from build123d import *

# Parameters (mm, degrees)
SKETCH1_W           = 152.4
SKETCH1_H           = 254
BOSS_EXTRUDE1_DEPTH = 6.35
CUT_EXTRUDE2_REACH  = 150.242
SKETCH3_R           = 2.5
CUT_EXTRUDE3_REACH  = 150.242
SKETCH4_R           = 2.75


with BuildPart() as part:
    # Sketch1 → Boss-Extrude1 (new body)
    with BuildSketch(Plane.XY):
        Rectangle(SKETCH1_W, SKETCH1_H)
    extrude(amount=BOSS_EXTRUDE1_DEPTH)

    # Sketch3 → Cut-Extrude2 (cut, up to next)
    with BuildSketch(Plane(origin=(0, 0, 0), x_dir=(-1, 0, 0), z_dir=(0, 0, -1)), mode=Mode.PRIVATE) as cut_extrude2_sk1:
        with Locations((63.7, -20.45)):
            Circle(SKETCH3_R)
    cut_extrude2_tool1 = extrude(cut_extrude2_sk1.sketch, amount=-CUT_EXTRUDE2_REACH, mode=Mode.PRIVATE) & part.part
    # Sketch3 → Cut-Extrude2 (cut, up to next)
    with BuildSketch(Plane(origin=(0, 0, 0), x_dir=(-1, 0, 0), z_dir=(0, 0, -1)), mode=Mode.PRIVATE) as cut_extrude2_sk2:
        with Locations((38.7, -20.45)):
            Circle(SKETCH3_R)
    cut_extrude2_tool2 = extrude(cut_extrude2_sk2.sketch, amount=-CUT_EXTRUDE2_REACH, mode=Mode.PRIVATE) & part.part
    # Sketch3 → Cut-Extrude2 (cut, up to next)
    with BuildSketch(Plane(origin=(0, 0, 0), x_dir=(-1, 0, 0), z_dir=(0, 0, -1)), mode=Mode.PRIVATE) as cut_extrude2_sk3:
        with Locations((38.7, -45.45)):
            Circle(SKETCH3_R)
    cut_extrude2_tool3 = extrude(cut_extrude2_sk3.sketch, amount=-CUT_EXTRUDE2_REACH, mode=Mode.PRIVATE) & part.part
    # Sketch3 → Cut-Extrude2 (cut, up to next)
    with BuildSketch(Plane(origin=(0, 0, 0), x_dir=(-1, 0, 0), z_dir=(0, 0, -1)), mode=Mode.PRIVATE) as cut_extrude2_sk4:
        with Locations((63.7, -45.45)):
            Circle(SKETCH3_R)
    cut_extrude2_tool4 = extrude(cut_extrude2_sk4.sketch, amount=-CUT_EXTRUDE2_REACH, mode=Mode.PRIVATE) & part.part
    # Sketch3 → Cut-Extrude2 (cut, up to next)
    with BuildSketch(Plane(origin=(0, 0, 0), x_dir=(-1, 0, 0), z_dir=(0, 0, -1)), mode=Mode.PRIVATE) as cut_extrude2_sk5:
        with Locations((63.7, -70.45)):
            Circle(SKETCH3_R)
    cut_extrude2_tool5 = extrude(cut_extrude2_sk5.sketch, amount=-CUT_EXTRUDE2_REACH, mode=Mode.PRIVATE) & part.part
    # Sketch3 → Cut-Extrude2 (cut, up to next)
    with BuildSketch(Plane(origin=(0, 0, 0), x_dir=(-1, 0, 0), z_dir=(0, 0, -1)), mode=Mode.PRIVATE) as cut_extrude2_sk6:
        with Locations((38.7, -70.45)):
            Circle(SKETCH3_R)
    cut_extrude2_tool6 = extrude(cut_extrude2_sk6.sketch, amount=-CUT_EXTRUDE2_REACH, mode=Mode.PRIVATE) & part.part
    # Sketch3 → Cut-Extrude2 (cut, up to next)
    with BuildSketch(Plane(origin=(0, 0, 0), x_dir=(-1, 0, 0), z_dir=(0, 0, -1)), mode=Mode.PRIVATE) as cut_extrude2_sk7:
        with Locations((38.7, -95.45)):
            Circle(SKETCH3_R)
    cut_extrude2_tool7 = extrude(cut_extrude2_sk7.sketch, amount=-CUT_EXTRUDE2_REACH, mode=Mode.PRIVATE) & part.part
    # Sketch3 → Cut-Extrude2 (cut, up to next)
    with BuildSketch(Plane(origin=(0, 0, 0), x_dir=(-1, 0, 0), z_dir=(0, 0, -1)), mode=Mode.PRIVATE) as cut_extrude2_sk8:
        with Locations((63.7, -95.45)):
            Circle(SKETCH3_R)
    cut_extrude2_tool8 = extrude(cut_extrude2_sk8.sketch, amount=-CUT_EXTRUDE2_REACH, mode=Mode.PRIVATE) & part.part
    # Sketch3 → Cut-Extrude2 (cut, up to next)
    with BuildSketch(Plane(origin=(0, 0, 0), x_dir=(-1, 0, 0), z_dir=(0, 0, -1)), mode=Mode.PRIVATE) as cut_extrude2_sk9:
        with Locations((-11.738, -61.16)):
            Circle(SKETCH3_R)
    cut_extrude2_tool9 = extrude(cut_extrude2_sk9.sketch, amount=-CUT_EXTRUDE2_REACH, mode=Mode.PRIVATE) & part.part
    # Sketch3 → Cut-Extrude2 (cut, up to next)
    with BuildSketch(Plane(origin=(0, 0, 0), x_dir=(-1, 0, 0), z_dir=(0, 0, -1)), mode=Mode.PRIVATE) as cut_extrude2_sk10:
        with Locations((-11.738, -36.16)):
            Circle(SKETCH3_R)
    cut_extrude2_tool10 = extrude(cut_extrude2_sk10.sketch, amount=-CUT_EXTRUDE2_REACH, mode=Mode.PRIVATE) & part.part
    # Sketch3 → Cut-Extrude2 (cut, up to next)
    with BuildSketch(Plane(origin=(0, 0, 0), x_dir=(-1, 0, 0), z_dir=(0, 0, -1)), mode=Mode.PRIVATE) as cut_extrude2_sk11:
        with Locations((-36.738, -61.16)):
            Circle(SKETCH3_R)
    cut_extrude2_tool11 = extrude(cut_extrude2_sk11.sketch, amount=-CUT_EXTRUDE2_REACH, mode=Mode.PRIVATE) & part.part
    # Sketch3 → Cut-Extrude2 (cut, up to next)
    with BuildSketch(Plane(origin=(0, 0, 0), x_dir=(-1, 0, 0), z_dir=(0, 0, -1)), mode=Mode.PRIVATE) as cut_extrude2_sk12:
        with Locations((-36.738, -36.16)):
            Circle(SKETCH3_R)
    cut_extrude2_tool12 = extrude(cut_extrude2_sk12.sketch, amount=-CUT_EXTRUDE2_REACH, mode=Mode.PRIVATE) & part.part
    # Sketch3 → Cut-Extrude2 (cut, up to next)
    with BuildSketch(Plane(origin=(0, 0, 0), x_dir=(-1, 0, 0), z_dir=(0, 0, -1)), mode=Mode.PRIVATE) as cut_extrude2_sk13:
        with Locations((-11.738, -11.16)):
            Circle(SKETCH3_R)
    cut_extrude2_tool13 = extrude(cut_extrude2_sk13.sketch, amount=-CUT_EXTRUDE2_REACH, mode=Mode.PRIVATE) & part.part
    # Sketch3 → Cut-Extrude2 (cut, up to next)
    with BuildSketch(Plane(origin=(0, 0, 0), x_dir=(-1, 0, 0), z_dir=(0, 0, -1)), mode=Mode.PRIVATE) as cut_extrude2_sk14:
        with Locations((-36.738, -11.16)):
            Circle(SKETCH3_R)
    cut_extrude2_tool14 = extrude(cut_extrude2_sk14.sketch, amount=-CUT_EXTRUDE2_REACH, mode=Mode.PRIVATE) & part.part
    # Sketch3 → Cut-Extrude2 (cut, up to next)
    with BuildSketch(Plane(origin=(0, 0, 0), x_dir=(-1, 0, 0), z_dir=(0, 0, -1)), mode=Mode.PRIVATE) as cut_extrude2_sk15:
        with Locations((-36.738, 13.84)):
            Circle(SKETCH3_R)
    cut_extrude2_tool15 = extrude(cut_extrude2_sk15.sketch, amount=-CUT_EXTRUDE2_REACH, mode=Mode.PRIVATE) & part.part
    # Sketch3 → Cut-Extrude2 (cut, up to next)
    with BuildSketch(Plane(origin=(0, 0, 0), x_dir=(-1, 0, 0), z_dir=(0, 0, -1)), mode=Mode.PRIVATE) as cut_extrude2_sk16:
        with Locations((-11.738, 13.84)):
            Circle(SKETCH3_R)
    cut_extrude2_tool16 = extrude(cut_extrude2_sk16.sketch, amount=-CUT_EXTRUDE2_REACH, mode=Mode.PRIVATE) & part.part
    add(cut_extrude2_tool1.solids().sort_by_distance((-63.7, -20.45, 0))[0], mode=Mode.SUBTRACT)
    add(cut_extrude2_tool2.solids().sort_by_distance((-38.7, -20.45, 0))[0], mode=Mode.SUBTRACT)
    add(cut_extrude2_tool3.solids().sort_by_distance((-38.7, -45.45, 0))[0], mode=Mode.SUBTRACT)
    add(cut_extrude2_tool4.solids().sort_by_distance((-63.7, -45.45, 0))[0], mode=Mode.SUBTRACT)
    add(cut_extrude2_tool5.solids().sort_by_distance((-63.7, -70.45, 0))[0], mode=Mode.SUBTRACT)
    add(cut_extrude2_tool6.solids().sort_by_distance((-38.7, -70.45, 0))[0], mode=Mode.SUBTRACT)
    add(cut_extrude2_tool7.solids().sort_by_distance((-38.7, -95.45, 0))[0], mode=Mode.SUBTRACT)
    add(cut_extrude2_tool8.solids().sort_by_distance((-63.7, -95.45, 0))[0], mode=Mode.SUBTRACT)
    add(cut_extrude2_tool9.solids().sort_by_distance((11.738, -61.16, 0))[0], mode=Mode.SUBTRACT)
    add(cut_extrude2_tool10.solids().sort_by_distance((11.738, -36.16, 0))[0], mode=Mode.SUBTRACT)
    add(cut_extrude2_tool11.solids().sort_by_distance((36.738, -61.16, 0))[0], mode=Mode.SUBTRACT)
    add(cut_extrude2_tool12.solids().sort_by_distance((36.738, -36.16, 0))[0], mode=Mode.SUBTRACT)
    add(cut_extrude2_tool13.solids().sort_by_distance((11.738, -11.16, 0))[0], mode=Mode.SUBTRACT)
    add(cut_extrude2_tool14.solids().sort_by_distance((36.738, -11.16, 0))[0], mode=Mode.SUBTRACT)
    add(cut_extrude2_tool15.solids().sort_by_distance((36.738, 13.84, 0))[0], mode=Mode.SUBTRACT)
    add(cut_extrude2_tool16.solids().sort_by_distance((11.738, 13.84, 0))[0], mode=Mode.SUBTRACT)

    # Sketch4 → Cut-Extrude3 (cut, up to next)
    with BuildSketch(Plane(origin=(0, 0, 0), x_dir=(-1, 0, 0), z_dir=(0, 0, -1)), mode=Mode.PRIVATE) as cut_extrude3_sk1:
        with Locations((-47.180499962, 58.762402402)):
            Circle(SKETCH4_R)
    cut_extrude3_tool1 = extrude(cut_extrude3_sk1.sketch, amount=-CUT_EXTRUDE3_REACH, mode=Mode.PRIVATE) & part.part
    # Sketch4 → Cut-Extrude3 (cut, up to next)
    with BuildSketch(Plane(origin=(0, 0, 0), x_dir=(-1, 0, 0), z_dir=(0, 0, -1)), mode=Mode.PRIVATE) as cut_extrude3_sk2:
        with Locations((-1.180499962, 58.762402402)):
            Circle(SKETCH4_R)
    cut_extrude3_tool2 = extrude(cut_extrude3_sk2.sketch, amount=-CUT_EXTRUDE3_REACH, mode=Mode.PRIVATE) & part.part
    # Sketch4 → Cut-Extrude3 (cut, up to next)
    with BuildSketch(Plane(origin=(0, 0, 0), x_dir=(-1, 0, 0), z_dir=(0, 0, -1)), mode=Mode.PRIVATE) as cut_extrude3_sk3:
        with Locations((-47.180499962, 76.762402402)):
            Circle(SKETCH4_R)
    cut_extrude3_tool3 = extrude(cut_extrude3_sk3.sketch, amount=-CUT_EXTRUDE3_REACH, mode=Mode.PRIVATE) & part.part
    # Sketch4 → Cut-Extrude3 (cut, up to next)
    with BuildSketch(Plane(origin=(0, 0, 0), x_dir=(-1, 0, 0), z_dir=(0, 0, -1)), mode=Mode.PRIVATE) as cut_extrude3_sk4:
        with Locations((-1.180499962, 76.762402402)):
            Circle(SKETCH4_R)
    cut_extrude3_tool4 = extrude(cut_extrude3_sk4.sketch, amount=-CUT_EXTRUDE3_REACH, mode=Mode.PRIVATE) & part.part
    add(cut_extrude3_tool1.solids().sort_by_distance((47.1805, 58.762402, 0))[0], mode=Mode.SUBTRACT)
    add(cut_extrude3_tool2.solids().sort_by_distance((1.1805, 58.762402, 0))[0], mode=Mode.SUBTRACT)
    add(cut_extrude3_tool3.solids().sort_by_distance((47.1805, 76.762402, 0))[0], mode=Mode.SUBTRACT)
    add(cut_extrude3_tool4.solids().sort_by_distance((1.1805, 76.762402, 0))[0], mode=Mode.SUBTRACT)


solid = part.part
Verification items for the finished model (mm, model axes). Coordinates: 2 decimals unless noted, no trailing zeros. Write each loop counter-clockwise with the first axis right and the second up, starting at its lowest first coordinate (ties: lowest second). Pieces come first, ordered by that corner, then holes. Notation, with made-up numbers: M 19,82 L 64,82 A24 ccw 64,101 Z; hole C 58,-14.5 d7. An arc over 180 degrees is marked long. One line per question, with ' | ' between items.
1) Release check for a two-part mould opening along Y. For faces 1 (the face through (-1, -127, 3)), 2 (the face through (-1, 127, 3)), 3 (the face through (-1, 2, 6.35)), 4 (the face through (10.394, -34.052, 3.131)) record: +Y half, -Y half, draft (parallel to the pull), parting line (faces both ways), or undercut.
Solutions:
face 1: -Y half | face 2: +Y half | face 3: draft | face 4: undercut
2) Material ranges on L1, parallel to X at y = -45.5, z = 5.75; L2, parallel to Y at x = -63.7, z = 2; L3, parallel to Y at x = -41, z = 2.75, recorded low to high.
Solutions:
L1: -76.2 to -66.2, -61.2 to -41.2, -36.2 to 76.2 | L2: -127 to -97.95, -92.95 to -72.95, -67.95 to -47.95, -42.95 to -22.95, -17.95 to 127 | L3: -127 to -96.43, -94.47 to -71.43, -69.47 to -46.43, -44.47 to -21.43, -19.47 to 127
3) Sectioned sample at A-A on y = -95.45. Record the cut outline in (x, z).
Solutions:
outline: M -76.2,0 L -66.2,0 L -66.2,6.35 L -76.2,6.35 Z; M -61.2,0 L -41.2,0 L -41.2,6.35 L -61.2,6.35 Z; M -36.2,0 L 76.2,0 L 76.2,6.35 L -36.2,6.35 Z
4) Sectioned sample at B-B on x = -38.7. Record the cut outline in (y, z).
Solutions:
outline: M -127,0 L -97.95,0 L -97.95,6.35 L -127,6.35 Z; M -92.95,0 L -72.95,0 L -72.95,6.35 L -92.95,6.35 Z; M -67.95,0 L -47.95,0 L -47.95,6.35 L -67.95,6.35 Z; M -42.95,0 L -22.95,0 L -22.95,6.35 L -42.95,6.35 Z; M -17.95,0 L 127,0 L 127,6.35 L -17.95,6.35 Z
